Source: CAD feature listing. Evaluate the final solid. Frame: model axes, mm. A direction names the side the tool comes from. Give positions to 0.01 mm unless a question says otherwise; leave off trailing zeros. Loops run counter-clockwise (first coordinate to the right, second up) from the corner with the lowest first, then second, coordinate; pieces in that order, holes last. Notation, with made-up numbers: (80, -0.5) -> (89, -0.5) arc R21 cw to (89, 23.5) -> close; hole circle Ø1 at (81.5, 8.5). An arc over 180 degrees is marked (long way). Return JSON: item names as keys, results as strings. Group by question number.
(1) Cut plane A-A on y = -6.75. Give the number of separate pieces and of enclosed holes in the cut face, then the cut area to 3 significant figures.
(2) Access query for faces 1 (the face through (34, -9, 0)), 2 (the face through (0, -3, 48)), 3 (the face through (14.1, 4.8, 22.7)), 4 (the face through (-10.5, -3, 24)), 5 (the face through (14, 10, 24)). Directions: +Z, -Z, +X, -X, +Y, -Y. A direction counts if a zero-diameter tool reaches every point of the face in a straight line with its end or side. Return the directions, or none.
(3) Cut plane B-B on z = 17. Return loops of the section in (x, y), then the cut area to 3 significant figures.
(4) Cut plane C-C on x = 31.5. Return loops of the section in (y, z), then the cut area to 3 significant figures.
(5) Ray query, line 1 (X direction, y = 0.25, z = 3); line 2 (Z direction, x = 14.5, y = 1.25); line 3 (Y direction, x = -1, z = 34). Return the intervals inside material, ascending. Write a range as from..to.
(6) Cut plane D-D on x = 22. Return loops of the section in (y, z).
(7) Pin query (flat end, axial travel): pin 1 (15 mm diameter, centred on x = 14.5, z = 26, fed in from -Y). Return the tip coordinate at first contact, or that it passes through.
```python
from build123d import *

# Parameters (mm, degrees)
BOX004_W          = 2
BOX004_H          = 12
BOX004_DEPTH      = 5
BOX005_W          = 2
BOX005_H          = 12
BOX005_DEPTH      = 5
BOX008_W          = 2
BOX008_H          = 12
BOX008_DEPTH      = 5
BOX003_W          = 2
BOX003_H          = 12
BOX003_DEPTH      = 5
BOX038_W          = 2
BOX038_H          = 12
BOX038_DEPTH      = 5
BOX028_W          = 2
BOX028_H          = 12
BOX028_DEPTH      = 5
BOX007_W          = 2
BOX007_H          = 12
BOX007_DEPTH      = 5
BOX039_W          = 2
BOX039_H          = 12
BOX039_DEPTH      = 5
BOX036_W          = 2.5
BOX036_H          = 12
BOX036_DEPTH      = 50
BOX037_W          = 2.5
BOX037_H          = 12
BOX037_DEPTH      = 50
BOX035_W          = 55
BOX035_H          = 12
BOX035_DEPTH      = 2.5
BOX034_W          = 55
BOX034_H          = 12
BOX034_DEPTH      = 2.5
CYLINDER066_R     = 1.65
CYLINDER066_DEPTH = 1.6
CYLINDER065_R     = 4.8
CYLINDER065_DEPTH = 42
CYLINDER068_R     = 1.65
CYLINDER068_DEPTH = 1.6
CYLINDER067_R     = 4.8
CYLINDER067_DEPTH = 42
CYLINDER070_R     = 1.65
CYLINDER070_DEPTH = 1.6
CYLINDER069_R     = 4.8
CYLINDER069_DEPTH = 42
CYLINDER072_R     = 1.65
CYLINDER072_DEPTH = 1.6
CYLINDER071_R     = 4.8
CYLINDER071_DEPTH = 42
CYLINDER074_R     = 1.65
CYLINDER074_DEPTH = 1.6
CYLINDER073_R     = 4.8
CYLINDER073_DEPTH = 42
BOX032_W          = 55
BOX032_H          = 7
BOX032_DEPTH      = 50


with BuildPart() as cube004:
    # Box004 → Box004 (new body)
    with BuildSketch(Plane(origin=(18.5, -9, 46), x_dir=(1, 0, 0), z_dir=(0, 0, 1))):
        with Locations((1, 6)):
            Rectangle(BOX004_W, BOX004_H)
    extrude(amount=BOX004_DEPTH)


with BuildPart() as cube005:
    # Box005 → Box005 (new body)
    with BuildSketch(Plane(origin=(-2, -9, 46), x_dir=(1, 0, 0), z_dir=(0, 0, 1))):
        with Locations((1, 6)):
            Rectangle(BOX005_W, BOX005_H)
    extrude(amount=BOX005_DEPTH)


with BuildPart() as cube008:
    # Box008 → Box008 (new body)
    with BuildSketch(Plane(origin=(8, -9, -2), x_dir=(1, 0, 0), z_dir=(0, 0, 1))):
        with Locations((1, 6)):
            Rectangle(BOX008_W, BOX008_H)
    extrude(amount=BOX008_DEPTH)


with BuildPart() as fusion107:
    # Box003 → Box003 (new body)
    with BuildSketch(Plane(origin=(28, -9, -2), x_dir=(1, 0, 0), z_dir=(0, 0, 1))):
        with Locations((1, 6)):
            Rectangle(BOX003_W, BOX003_H)
    extrude(amount=BOX003_DEPTH)

    # Fusion107: union Cube004, Cube005, Cube008
    add(cube004.part)
    add(cube005.part)
    add(cube008.part)


with BuildPart() as cube036:
    # Box038 → Box038 (new body)
    with BuildSketch(Plane(origin=(-10.5, -9, 46), x_dir=(1, 0, 0), z_dir=(0, 0, 1))):
        with Locations((1, 6)):
            Rectangle(BOX038_W, BOX038_H)
    extrude(amount=BOX038_DEPTH)


with BuildPart() as cube027:
    # Box028 → Box028 (new body)
    with BuildSketch(Plane(origin=(37.5, -9, -2), x_dir=(1, 0, 0), z_dir=(0, 0, 1))):
        with Locations((1, 6)):
            Rectangle(BOX028_W, BOX028_H)
    extrude(amount=BOX028_DEPTH)


with BuildPart() as cube007:
    # Box007 → Box007 (new body)
    with BuildSketch(Plane(origin=(37.5, -9, 46), x_dir=(1, 0, 0), z_dir=(0, 0, 1))):
        with Locations((1, 6)):
            Rectangle(BOX007_W, BOX007_H)
    extrude(amount=BOX007_DEPTH)


with BuildPart() as fusion106:
    # Box039 → Box039 (new body)
    with BuildSketch(Plane(origin=(-10.5, -9, -2), x_dir=(1, 0, 0), z_dir=(0, 0, 1))):
        with Locations((1, 6)):
            Rectangle(BOX039_W, BOX039_H)
    extrude(amount=BOX039_DEPTH)

    # Fusion106: union Cube036, Cube027, Cube007
    add(cube036.part)
    add(cube027.part)
    add(cube007.part)


with BuildPart() as cube034:
    # Box036 → Box036 (new body)
    with BuildSketch(Plane(origin=(-13, -9, -1), x_dir=(1, 0, 0), z_dir=(0, 0, 1))):
        with Locations((1.25, 6)):
            Rectangle(BOX036_W, BOX036_H)
    extrude(amount=BOX036_DEPTH)


with BuildPart() as cube035:
    # Box037 → Box037 (new body)
    with BuildSketch(Plane(origin=(39.5, -9, -1), x_dir=(1, 0, 0), z_dir=(0, 0, 1))):
        with Locations((1.25, 6)):
            Rectangle(BOX037_W, BOX037_H)
    extrude(amount=BOX037_DEPTH)


with BuildPart() as cube033:
    # Box035 → Box035 (new body)
    with BuildSketch(Plane(origin=(-13, -9, 46.5), x_dir=(1, 0, 0), z_dir=(0, 0, 1))):
        with Locations((27.5, 6)):
            Rectangle(BOX035_W, BOX035_H)
    extrude(amount=BOX035_DEPTH)


with BuildPart() as cut045024:
    # Box034 → Box034 (new body)
    with BuildSketch(Plane(origin=(-13, -9, -1), x_dir=(1, 0, 0), z_dir=(0, 0, 1))):
        with Locations((27.5, 6)):
            Rectangle(BOX034_W, BOX034_H)
    extrude(amount=BOX034_DEPTH)

    # Fusion105: union Cube034, Cube035, Cube033
    add(cube034.part)
    add(cube035.part)
    add(cube033.part)

    # Cut045023: cut Fusion106
    add(fusion106.part, mode=Mode.SUBTRACT)

    # Cut045024: cut Fusion107
    add(fusion107.part, mode=Mode.SUBTRACT)


with BuildPart() as cylinder118:
    # Cylinder066 → Cylinder066 (new body)
    with BuildSketch(Plane.XY.offset(42)):
        Circle(CYLINDER066_R)
    extrude(amount=CYLINDER066_DEPTH)


with BuildPart() as fusion097:
    # Cylinder065 → Cylinder065 (new body)
    with BuildSketch(Plane.XY):
        Circle(CYLINDER065_R)
    extrude(amount=CYLINDER065_DEPTH)

    # Fusion097: union Cylinder118
    add(cylinder118.part)


with BuildPart() as fusion097_1:
    # Fusion097 placement: moved
    add(fusion097.part.moved(Location((2, 0, 0))))


with BuildPart() as cylinder120:
    # Cylinder068 → Cylinder068 (new body)
    with BuildSketch(Plane.XY.offset(42)):
        Circle(CYLINDER068_R)
    extrude(amount=CYLINDER068_DEPTH)


with BuildPart() as fusion098:
    # Cylinder067 → Cylinder067 (new body)
    with BuildSketch(Plane.XY):
        Circle(CYLINDER067_R)
    extrude(amount=CYLINDER067_DEPTH)

    # Fusion098: union Cylinder120
    add(cylinder120.part)


with BuildPart() as fusion098_1:
    # Fusion098 placement: moved
    add(fusion098.part.moved(Location((12, 0, 0))))


with BuildPart() as cylinder122:
    # Cylinder070 → Cylinder070 (new body)
    with BuildSketch(Plane.XY.offset(42)):
        Circle(CYLINDER070_R)
    extrude(amount=CYLINDER070_DEPTH)


with BuildPart() as fusion099:
    # Cylinder069 → Cylinder069 (new body)
    with BuildSketch(Plane.XY):
        Circle(CYLINDER069_R)
    extrude(amount=CYLINDER069_DEPTH)

    # Fusion099: union Cylinder122
    add(cylinder122.part)


with BuildPart() as fusion099_1:
    # Fusion099 placement: moved
    add(fusion099.part.moved(Location((22, 0, 0))))


with BuildPart() as cylinder124:
    # Cylinder072 → Cylinder072 (new body)
    with BuildSketch(Plane.XY.offset(42)):
        Circle(CYLINDER072_R)
    extrude(amount=CYLINDER072_DEPTH)


with BuildPart() as fusion100:
    # Cylinder071 → Cylinder071 (new body)
    with BuildSketch(Plane.XY):
        Circle(CYLINDER071_R)
    extrude(amount=CYLINDER071_DEPTH)

    # Fusion100: union Cylinder124
    add(cylinder124.part)


with BuildPart() as fusion100_1:
    # Fusion100 placement: moved
    add(fusion100.part.moved(Location((32, 0, 0))))


with BuildPart() as cylinder126:
    # Cylinder074 → Cylinder074 (new body)
    with BuildSketch(Plane.XY.offset(42)):
        Circle(CYLINDER074_R)
    extrude(amount=CYLINDER074_DEPTH)


with BuildPart() as aaa_batts001:
    # Cylinder073 → Cylinder073 (new body)
    with BuildSketch(Plane.XY):
        Circle(CYLINDER073_R)
    extrude(amount=CYLINDER073_DEPTH)

    # Fusion101: union Cylinder126
    add(cylinder126.part)


with BuildPart() as aaa_batts001_1:
    # Fusion101 placement: moved
    add(aaa_batts001.part.moved(Location((-8, 0, 0))))

    # Fusion102: union Fusion097, Fusion098, Fusion099, Fusion100
    add(fusion097_1.part)
    add(fusion098_1.part)
    add(fusion099_1.part)
    add(fusion100_1.part)


with BuildPart() as aaa_batts001_2:
    # Fusion102 placement: moved
    add(aaa_batts001_1.part.moved(Location((2, 0, 2))))


with BuildPart() as fusion110:
    # Box032 → Box032 (new body)
    with BuildSketch(Plane(origin=(-13, 3, -1), x_dir=(1, 0, 0), z_dir=(0, 0, 1))):
        with Locations((27.5, 3.5)):
            Rectangle(BOX032_W, BOX032_H)
    extrude(amount=BOX032_DEPTH)

    # Cut045022: cut AAA Batts001
    add(aaa_batts001_2.part, mode=Mode.SUBTRACT)

    # Fusion110: union Cut045024
    add(cut045024.part)


solid = fusion110.part
```
Answers:
{
 "1": {"separate pieces": "8", "enclosed holes": "0", "area": "460 mm²"},
 "2": {"face 1": "+Z, -Z, +X, -X, -Y", "face 2": "+Z, -Y", "face 3": "-Y", "face 4": "+Z, -Z, -Y", "face 5": "+Z, -Z, +X, -X, +Y"},
 "3": {"outline": "(-13, -9) -> (-10.5, -9) -> (-10.5, 3) -> (-9.75, 3) arc R4.8 cw to (-2.25, 3) -> (0.25, 3) arc R4.8 cw to (7.75, 3) -> (10.25, 3) arc R4.8 cw to (17.75, 3) -> (20.25, 3) arc R4.8 cw to (27.75, 3) -> (30.25, 3) arc R4.8 cw to (37.75, 3) -> (39.5, 3) -> (39.5, -9) -> (42, -9) -> (42, 10) -> (-13, 10) -> close", "area": "398 mm²"},
 "4": {"outline": "(-9, -1) -> (10, -1) -> (10, 49) -> (-9, 49) -> (-9, 46.5) -> (3, 46.5) -> (3, 44) -> (4.1, 44) -> (4.1, 2) -> (3, 2) -> (3, 1.5) -> (-9, 1.5) -> close", "area": "364 mm²"},
 "5": {"line 1": "-13..-10.5, 39.5..42", "line 2": "-1..1.5, 46.5..49", "line 3": "3..10"},
 "6": {"outline": "(-9, -1) -> (10, -1) -> (10, 49) -> (-9, 49) -> (-9, 46.5) -> (3, 46.5) -> (3, 44) -> (4.36, 44) -> (4.36, 2) -> (3, 2) -> (3, 1.5) -> (-9, 1.5) -> close"},
 "7": {"pin 1": "y = 3"}
}
